```python
from build123d import *

# Parameters (mm, degrees)
BOSS_EXTRUDE1_DEPTH = 34.5
FILLET1_R           = 1
SKETCH2_R           = 1
CUT_EXTRUDE1_DEPTH  = 496.614236654


with BuildPart() as part:
    # Sketch1 → Boss-Extrude1 (new body)
    with BuildSketch(Plane.XY.offset(40)):
        with BuildLine():
            Line((-312.030492528, 377.868524993), (-310.193868717, 375.244776692))
            Line((-310.193868717, 375.244776692), (-310.096008301, 367.875213623))
            Line((-310.096008301, 367.875213623), (-311.889068604, 365.166412354))
            Line((-311.889068604, 365.166412354), (-314.88168335, 362.936676025))
            Line((-314.88168335, 362.936676025), (-314.88168335, 347.918438133))
            Line((-314.88168335, 347.918438133), (-302.847373473, 347.918438133))
            Line((-302.847373473, 347.918438133), (-302.847373473, 367.04556325))
            Line((-302.847373473, 367.04556325), (-304.028060208, 373.263846724))
            Line((-304.028060208, 373.263846724), (-306.153296332, 377.278181625))
            Line((-306.153296332, 377.278181625), (-308.864528411, 380.917030307))
            ThreePointArc((-308.864528411, 380.917030307), (-311.535911341, 380.523114569), (-312.030492528, 377.868524993))
        make_face()
        with BuildLine():
            Line((-312.988408734, 360.598376943), (-312.988408734, 353.109979303))
            Line((-312.988408734, 353.109979303), (-305, 352.927314193))
            Line((-305, 352.927314193), (-305, 365))
            Line((-305, 365), (-305.952850342, 371.670013428))
            ThreePointArc((-305.952850342, 371.670013428), (-306.959348498, 372.584855641), (-307.99460106, 371.702683918))
            Line((-307.99460106, 371.702683918), (-307.99460106, 366.023339102))
            Line((-307.99460106, 366.023339102), (-312.988408734, 360.598376943))
        make_face(mode=Mode.SUBTRACT)
    extrude(amount=BOSS_EXTRUDE1_DEPTH)

    # Fillet1
    fillet1_edges = [part.edges().sort_by_distance(p)[0] for p in [
        (-302.847373473, 347.918438133, 57.25),
        (-314.88168335, 347.918438133, 57.25),
        (-314.88168335, 362.936676025, 57.25),
        (-307.99460106, 366.023339102, 57.25),
        (-312.988408734, 360.598376943, 57.25),
        (-312.988408734, 353.109979303, 57.25),
        (-305, 352.927314193, 57.25),
    ]]
    fillet(fillet1_edges, radius=FILLET1_R)

    # Sketch2 → Cut-Extrude1 (cut, through all)
    with BuildSketch(Plane.XY.offset(74.5)):
        with Locations((-313.031111026, 350.560286037)):
            Circle(SKETCH2_R)
        with Locations((-304.91451991, 350.560286037)):
            Circle(SKETCH2_R)
    extrude(amount=-CUT_EXTRUDE1_DEPTH, mode=Mode.SUBTRACT)


solid = part.part
```
Work out the finished part from the listing and answer in its coordinate system (mm). A direction names the side the tool comes from. Give positions to 0.01 mm unless a question says otherwise; leave off trailing zeros. Order: outer loops, then holes, each group sorted by start corner. A loop starts at its lowest first (then second) coordinate and runs counter-clockwise, first axis right, second up.
1. For faces 5 (the flat face through (-311.13, 376.58, 57.01)), 6 (the cylindrical face through (-312.711, 353.396, 57.492)), 7 (the flat face through (-310, 365, 74.5)), determine the directions among +Z, -Z, +X, -X, +Y, -Y from which every point of the face is accessible in a straight line to the end or side of a thin tool.
Result sheet:
face 5: +Z, -Z, -X
face 6: +Z, -Z
face 7: +Z, +X, -X, +Y, -Y
2. Each of these flat-tipped pins is pushed along its axis until it touches: P1, Ø1.6, axis at x = -313.03, y = 350.56, coming from the -Z side; P2, Ø1.5, axis at x = -306.5, z = 71, coming from the +Y side; P3, Ø1.6, axis at y = 369.5, z = 62.5, coming from the +X side; P4, Ø2, axis at x = -313, z = 57, coming from the +Y side. Where does it stop, or does it pass through?
Result sheet:
P1: passes through
P2: stops at y = 378.75
P3: stops at x = -303.16
P4: stops at y = 379.89
3. Section A-A, the plane x = -307.5 is taken. Determine the outline of the cut face in (y, z), and give its area (3 significant figures).
Result sheet:
outline: (347.92, 40) - (352.98, 40) - (352.98, 74.5) - (347.92, 74.5) - close; (372.44, 40) - (379.09, 40) - (379.09, 74.5) - (372.44, 74.5) - close
area: 404 mm2
4. Section D-D, the plane z = 51.5 is taken. Determine the outline of the cut face in (x, y).
Result sheet:
outline: (-314.88, 348.92) arc R1 ccw to (-313.88, 347.92) - (-303.85, 347.92) arc R1 ccw to (-302.85, 348.92) - (-302.85, 367.05) - (-304.03, 373.26) - (-306.15, 377.28) - (-308.86, 380.92) arc R2.32 ccw to (-312.03, 377.87) - (-310.19, 375.24) - (-310.1, 367.88) - (-311.89, 365.17) - (-314.48, 363.24) arc R1 ccw to (-314.88, 362.43) - close; hole circle Ø2 at (-313.03, 350.56); hole (-312.99, 354.09) arc R1 ccw to (-312.01, 353.09) - (-306.02, 352.95) arc R1 ccw to (-305, 353.95) - (-305, 365) - (-305.95, 371.67) arc R1.03 ccw to (-307.99, 371.7) - (-307.99, 366.41) arc R1 cw to (-308.26, 365.74) - (-312.72, 360.89) arc R1 ccw to (-312.99, 360.21) - close; hole circle Ø2 at (-304.91, 350.56)
5. Straight lines are drawn through the part: L1, parallel to X at y = 356, z = 46; L2, parallel to Y at x = -308.25, z = 52.5; L3, parallel to X at y = 366.5, z = 66. For each, find the intervals that lie inside material, in ascending order.
Result sheet:
L1: x = -314.88 to -312.99, -305 to -302.85
L2: y = 347.92 to 353, 365.75 to 380.09
L3: x = -311.01 to -307.99, -305.21 to -302.85
6. The mould has two halves that part along X. Classify faces 1 (the cylindrical face through (-314.77, 362.89, 57.49)), 2 (the cylindrical face through (-311.51, 380.55, 57.01)), 3 (the flat face through (-307.995, 369, 57)), 4 (the flat face through (-309, 347.918, 57)): released by +X, released by -X, zero draft, split by the parting line, or undercut.
Result sheet:
face 1: released by -X
face 2: split by the parting line
face 3: undercut
face 4: zero draft
7. Section B-B, the plane y = 370 is taken. Determine the outline of the cut face in (x, z), and give its area (3 significant figures).
Result sheet:
outline: (-310.12, 40) - (-307.99, 40) - (-307.99, 74.5) - (-310.12, 74.5) - close; (-305.71, 40) - (-303.41, 40) - (-303.41, 74.5) - (-305.71, 74.5) - close
area: 153 mm2
8. Section C-C, the plane x = -305.5 is taken. Determine the outline of the cut face in (y, z).
Result sheet:
outline: (347.92, 40) - (349.75, 40) - (349.75, 74.5) - (347.92, 74.5) - close; (351.37, 40) - (353.08, 40) - (353.08, 74.5) - (351.37, 74.5) - close; (368.5, 40) - (376.04, 40) - (376.04, 74.5) - (368.5, 74.5) - close
